from build123d import *

# Parameters (mm, degrees)
BOSS_EXTRUDE1_DEPTH = 12
BOSS_EXTRUDE2_DEPTH = 4
SKETCH3_R           = 2.5
BOSS_EXTRUDE3_DEPTH = 3


with BuildPart() as part:
    # Sketch1 → Boss-Extrude1 (new body)
    with BuildSketch(Plane.XY):
        Polygon((0, 0), (0, 16.5), (4.5, 16.5), (4.5, 19), (0, 19), (0, 23), (-22.6, 23), (-22.6, 19), (-27.1, 19), (-27.1, 16.5), (-22.6, 16.5), (-22.6, 0), align=None)
    extrude(amount=BOSS_EXTRUDE1_DEPTH)

    # Sketch2 → Boss-Extrude2 (add)
    with BuildSketch(Plane(origin=(0, 23, 0), x_dir=(1, 0, 0), z_dir=(0, 1, 0))):
        with BuildLine():
            ThreePointArc((-6, 0), (-12, -6), (-6, -12))
            Line((-6, -12), (-6, 0))
        make_face()
        with BuildLine():
            Line((-6, 0), (-6, -12))
            ThreePointArc((-6, -12), (-1.757359313, -10.242640687), (0, -6))
            ThreePointArc((0, -6), (-1.757359313, -1.757359313), (-6, 0))
        make_face()
    extrude(amount=BOSS_EXTRUDE2_DEPTH)

    # Sketch3 → Boss-Extrude3 (add)
    with BuildSketch(Plane(origin=(0, 27, 0), x_dir=(1, 0, 0), z_dir=(0, 1, 0))):
        with Locations(Location((-6, -6, 0), (0, 0, 180))):
            Circle(SKETCH3_R)
    extrude(amount=BOSS_EXTRUDE3_DEPTH)


solid = part.part
Check sheet for the modelled part. Datum: model origin and axes. Units: mm. A direction names the side the tool comes from. Round coordinates to 2 decimals unless told otherwise and drop trailing zeros. Order: outer loops, then holes, each group sorted by start corner. A loop starts at its lowest first (then second) coordinate and runs counter-clockwise, first axis right, second up.
Q1. Scan lines: L1, parallel to X at y = 4.25, z = 5.5; L2, parallel to Y at x = -7, z = 11; L3, parallel to Y at x = -19, z = 7. Record each from-to range of solid material in increasing order.
Filled sheet:
L1: x = -22.6 to 0
L2: y = 0 to 27
L3: y = 0 to 23
Q2. Depth check by flat-ended pin: P1, Ø1.3, axis at x = -24.5, z = 9, coming from the -Y side; P2, Ø1, axis at x = -12, y = 25, coming from the -Z side; P3, Ø6, axis at y = 5.5, z = 5, coming from the -X side. Enter the tip coordinate at first touch or a pass-through.
Filled sheet:
P1: stops at y = 16.5
P2: stops at z = 3.6
P3: stops at x = -22.6
Q3. Cross-section at A-A, the plane z = 7.5. Enter the section's corners in (x, y).
Filled sheet:
outline: (-27.1, 16.5) - (-22.6, 16.5) - (-22.6, 0) - (0, 0) - (0, 16.5) - (4.5, 16.5) - (4.5, 19) - (0, 19) - (0, 23) - (-0.19, 23) - (-0.19, 27) - (-4, 27) - (-4, 30) - (-8, 30) - (-8, 27) - (-11.81, 27) - (-11.81, 23) - (-22.6, 23) - (-22.6, 19) - (-27.1, 19) - close
Q4. Cross-section at C-C, the plane z = 5. Enter the section's corners in (x, y), plus the area to 3 significant figures.
Filled sheet:
outline: (-27.1, 16.5) - (-22.6, 16.5) - (-22.6, 0) - (0, 0) - (0, 16.5) - (4.5, 16.5) - (4.5, 19) - (0, 19) - (0, 23) - (-0.08, 23) - (-0.08, 27) - (-3.71, 27) - (-3.71, 30) - (-8.29, 30) - (-8.29, 27) - (-11.92, 27) - (-11.92, 23) - (-22.6, 23) - (-22.6, 19) - (-27.1, 19) - close
area: 603 mm2
Q5. Set-up check for faces 1 (the face through (2, 19, 6)), 2 (the face through (-1, 23, 1)), 3 (the face through (2, 16.5, 6)): record each of +Z, -Z, +X, -X, +Y, -Y from which the full face is reachable in a straight line by a thin tool's end or side.
Filled sheet:
face 1: +Z, -Z, +X, +Y
face 2: -Z, +X, +Y
face 3: +Z, -Z, +X, -Y
Q6. Cross-section at B-B, the plane y = 15. Enter the section's corners in (x, z), plus the area to 3 significant figures.
Filled sheet:
outline: (-22.6, 0) - (0, 0) - (0, 12) - (-22.6, 12) - close
area: 271 mm2
